Job drawing, mm, ordinate dimensions from the low corner. One solid piece. Give positions to 0.01 mm unless a question says otherwise; leave off trailing zeros. Write each loop counter-clockwise with the first axis right and the second up, starting at its lowest first coordinate (ties: lowest second). Pieces come first, ordered by that corner, then holes. Notation, with made-up numbers: M 62.5,59 L 80.5,59 A19 cw 80.5,90 Z; hole C 52,-11 d2. An arc over 180 degrees is marked long. Use CSV: the item, a comma, the result in double quotes. Start each with the question number.
Item 1: Pin check, flat tips, straight feed: pin 1 (2 mm diameter, centred on x = 47, z = 2, fed in from -Y); pin 2 (2 mm diameter, centred on x = 66, z = 2, fed in from -Y); pin 3 (2 mm diameter, centred on x = 52, y = 40.5, fed in from -Z). Stop position of each tip, or through.
Item 2: Cut at D-D (x = 86.01). List the corners of the cut face in (y, z).
Item 3: Cut at B-B (x = 61). List the corners of the cut face in (y, z).
Item 4: Cut at C-C (x = 71.16). List the corners of the cut face in (y, z), then the cut area to 3 significant figures.
Item 5: Cut at A-A (z = 2). Count the separate pieces of the cut face and the enclosed holes in it, then the cut area to 3 significant figures.
Item 6: Drill centre lines: line 1 (X direction, y = 53.22, z = 1.4); line 2 (X direction, y = 8.75, z = 2) (3 decimals); line 3 (Y direction, x = 71.16, z = 2.15). Where is each one in solid material? Low to high. Write a range as [from, to].
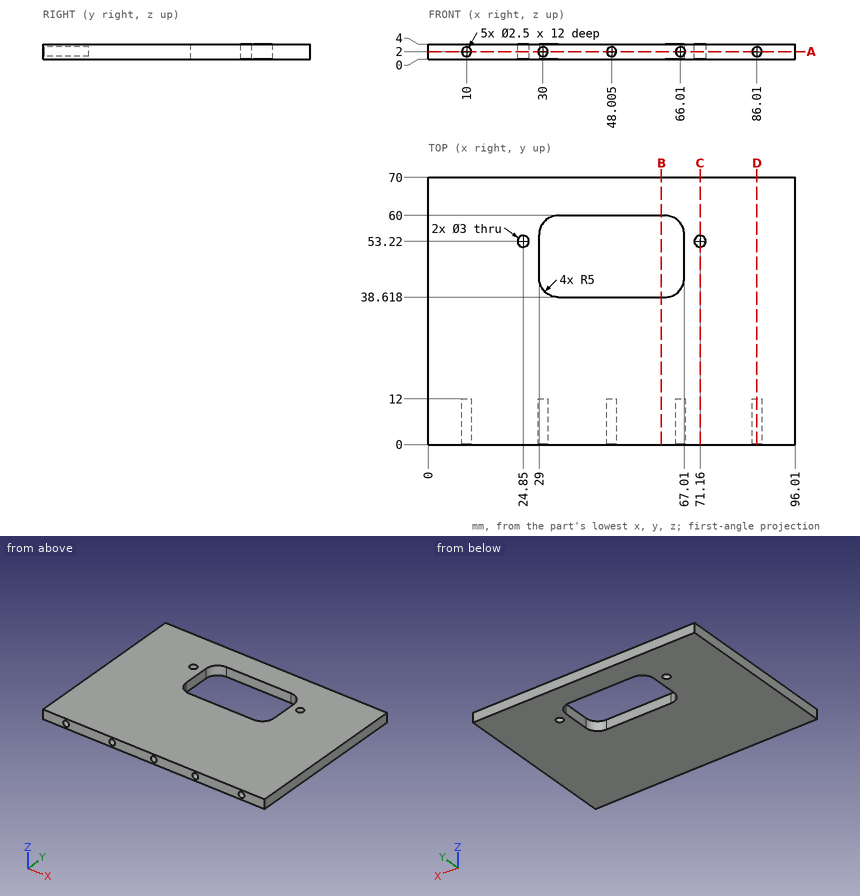
Worked answers:
1,pin 1,"stops at y = 0"
1,pin 2,"stops at y = 12"
1,pin 3,"passes through"
2,outline,"M 0,0 L 70,0 L 70,4 L 0,4 L 0,3.25 L 12,3.25 L 12,0.75 L 0,0.75 Z"
3,outline,"M 0,0 L 38.62,0 L 38.62,4 L 0,4 Z; M 60,0 L 70,0 L 70,4 L 60,4 Z"
4,outline,"M 0,0 L 51.72,0 L 51.72,4 L 0,4 Z; M 54.72,0 L 70,0 L 70,4 L 54.72,4 Z"
4,area,"268 mm^2"
5,separate pieces,"1"
5,enclosed holes,"3"
5,area,"5,770 mm^2"
6,line 1,"x = [0, 23.35], [26.35, 29], [67.01, 69.66], [72.66, 96.01]"
6,line 2,"x = [0, 8.75], [11.25, 28.75], [31.25, 46.755], [49.255, 64.76], [67.26, 84.76], [87.26, 96.01]"
6,line 3,"y = [0, 51.72], [54.72, 70]"
